Work out the finished part from the listing and answer in its coordinate system (mm). Round coordinates to 2 decimals unless told otherwise and drop trailing zeros. Write each loop counter-clockwise with the first axis right and the second up, starting at its lowest first coordinate (ties: lowest second). Pieces come first, ordered by that corner, then holes.
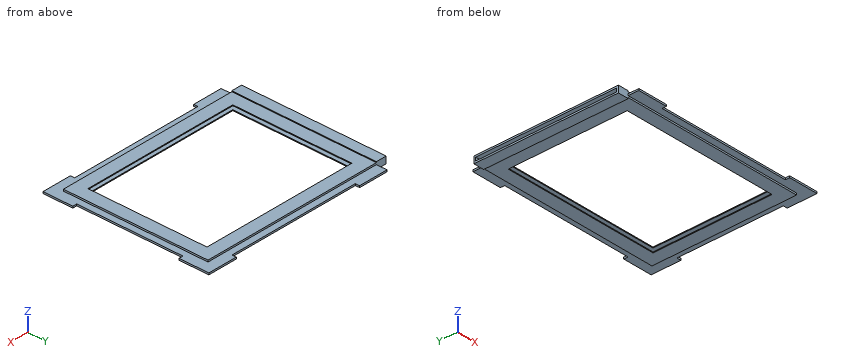
from build123d import *

# Parameters (mm, degrees)
F0_W     = 215
F0_H     = 170
F0_W_2   = 185
F0_H_2   = 140
F1_DEPTH = 3
F0_W_3   = 12.5
F2_DEPTH = 4
F3_DEPTH = 1
F4_W     = 166
F4_H     = 4
F5_DEPTH = 225.5


with BuildPart() as f1:
    # F0 (on Top) → F1 (new body, symmetric)
    with BuildSketch(Plane.XY):
        Rectangle(F0_W, F0_H)
        Rectangle(F0_W_2, F0_H_2, mode=Mode.SUBTRACT)
    extrude(amount=F1_DEPTH, both=True)

    # F0 (on Top) → F2 (join, symmetric)
    with BuildSketch(Plane.XY):
        with Locations((-113.75, 0)):
            Rectangle(F0_W_3, F0_H)
    extrude(amount=F2_DEPTH, both=True)

    # F0 (on Top) → F3 (join, symmetric)
    with BuildSketch(Plane.XY):
        Polygon((120, 62.5), (120, 97.5), (85, 97.5), (85, 92.5), (-72.5, 92.5), (-72.5, 97.5), (-107.5, 97.5), (-107.5, 85), (107.5, 85), (107.5, -85), (-107.5, -85), (-107.5, -97.5), (-72.5, -97.5), (-72.5, -92.5), (85, -92.5), (85, -97.5), (120, -97.5), (120, -62.5), (115, -62.5), (115, 62.5), align=None)
    extrude(amount=F3_DEPTH, both=True)

    # F4 (on face) → F5 (cut)
    with BuildSketch(Plane(origin=(-120, 0, 0), x_dir=(0, -1, 0), z_dir=(-1, 0, 0))):
        Rectangle(F4_W, F4_H)
    extrude(amount=-F5_DEPTH, mode=Mode.SUBTRACT)


solid = f1.part
Q1. Find section A-A (y = -65). Determine the outline of the cut face in (x, z), plus the area to 3 significant figures.
Q2. Find section D-D (y = 31). Determine the outline of the cut face in (x, z), plus the area to 3 significant figures.
Q3. Find the intervals of material crossed by L1, parallel to Y at x = 12.5, z = 0; L2, parallel to X at y = 58, z = 2.5; L3, parallel to Z at x = -109, y = 6, in increasing order.
Q4. Find section C-C (x = 99). Determine the outline of the cut face in (y, z).
Q5. Given pin 1 (0.5 mm diameter, centred on x = -29.5, z = -2.5, fed in from -Y); pin 2 (3 mm diameter, centred on x = -60, z = 0, fed in from +Y); pin 3 (1.5 mm diameter, centred on x = 70.5, z = 1, fed in from -Y), each flat-ended and moving along its own axis, determine where each tip first touches the part or whether it passes through.
Q6. Find section B-B (x = 50.5). Determine the outline of the cut face in (y, z), plus the area to 3 significant figures.
Report:
1. outline: (-120, -4) - (-107.5, -4) - (-107.5, -3) - (-92.5, -3) - (-92.5, -2) - (-120, -2) - close; (-120, 2) - (-92.5, 2) - (-92.5, 3) - (-107.5, 3) - (-107.5, 4) - (-120, 4) - close; (92.5, -3) - (107.5, -3) - (107.5, -1) - (120, -1) - (120, 1) - (107.5, 1) - (107.5, 3) - (92.5, 3) - (92.5, 2) - (105.5, 2) - (105.5, -2) - (92.5, -2) - close
1. area: 143 mm2
2. outline: (-120, -4) - (-107.5, -4) - (-107.5, -3) - (-92.5, -3) - (-92.5, -2) - (-120, -2) - close; (-120, 2) - (-92.5, 2) - (-92.5, 3) - (-107.5, 3) - (-107.5, 4) - (-120, 4) - close; (92.5, -3) - (107.5, -3) - (107.5, -1) - (115, -1) - (115, 1) - (107.5, 1) - (107.5, 3) - (92.5, 3) - (92.5, 2) - (105.5, 2) - (105.5, -2) - (92.5, -2) - close
2. area: 133 mm2
3. L1: y = -92.5 to -83, 83 to 92.5
3. L2: x = -120 to -92.5, 92.5 to 107.5
3. L3: z = -4 to -2, 2 to 4
4. outline: (-97.5, -1) - (-85, -1) - (-85, -3) - (85, -3) - (85, -1) - (97.5, -1) - (97.5, 1) - (85, 1) - (85, 3) - (-85, 3) - (-85, 1) - (-97.5, 1) - close; hole (-83, -2) - (83, -2) - (83, 2) - (-83, 2) - close
5. pin 1: stops at y = -85
5. pin 2: stops at y = 92.5
5. pin 3: stops at y = -92.5
6. outline: (-92.5, -1) - (-85, -1) - (-85, -3) - (-70, -3) - (-70, -2) - (-83, -2) - (-83, 2) - (-70, 2) - (-70, 3) - (-85, 3) - (-85, 1) - (-92.5, 1) - close; (70, -3) - (85, -3) - (85, -1) - (92.5, -1) - (92.5, 1) - (85, 1) - (85, 3) - (70, 3) - (70, 2) - (83, 2) - (83, -2) - (70, -2) - close
6. area: 106 mm2
